from build123d import *

# Parameters (mm, degrees)
BOSS_EXTRUDE2_DEPTH = 3.175
SKETCH4_W           = 28.575
SKETCH4_H           = 79.375
CUT_EXTRUDE2_DEPTH  = 3.175
CUT_EXTRUDE3_DEPTH  = 3.175
SKETCH9_R           = 3.175
CUT_EXTRUDE4_DEPTH  = 3.175
SKETCH11_W          = 25.4
SKETCH11_H          = 3.175
BOSS_EXTRUDE3_DEPTH = 12.7
FILLET2_R           = 3.175


with BuildPart() as part:
    # Sketch1 → Boss-Extrude2 (new body)
    with BuildSketch(Plane.XY):
        Polygon((0, 298.45), (25.4, 323.85), (279.4, 323.85), (304.8, 298.45), (304.8, 25.4), (279.4, 0), (25.4, 0), (0, 25.4), align=None)
    extrude(amount=BOSS_EXTRUDE2_DEPTH)

    # Sketch4 → Cut-Extrude2 (cut)
    with BuildSketch(Plane.XY.offset(3.175)):
        with Locations((14.2875, 161.925)):
            Rectangle(SKETCH4_W, SKETCH4_H)
    extrude(amount=-CUT_EXTRUDE2_DEPTH, mode=Mode.SUBTRACT)

    # Sketch5 → Cut-Extrude3 (cut)
    with BuildSketch(Plane.XY.offset(3.175)):
        with BuildLine():
            Line((98.425, 275.149783319), (247.65, 275.149783319))
            ThreePointArc((247.65, 275.149783319), (270.100640303, 265.850423621), (279.4, 243.399783319))
            Line((279.4, 243.399783319), (279.4, 207.424891659))
            ThreePointArc((279.4, 207.424891659), (270.100640303, 184.974251357), (247.65, 175.674891659))
            Line((247.65, 175.674891659), (98.425, 175.674891659))
            ThreePointArc((98.425, 175.674891659), (75.974359697, 184.974251357), (66.675, 207.424891659))
            Line((66.675, 207.424891659), (66.675, 243.399783319))
            ThreePointArc((66.675, 243.399783319), (75.974359697, 265.850423621), (98.425, 275.149783319))
        make_face()
        with BuildLine():
            Line((98.425, 150.274891659), (247.65, 150.274891659))
            ThreePointArc((247.65, 150.274891659), (270.100640303, 140.975531962), (279.4, 118.524891659))
            Line((279.4, 118.524891659), (279.4, 82.55))
            ThreePointArc((279.4, 82.55), (270.100640303, 60.099359697), (247.65, 50.8))
            Line((247.65, 50.8), (98.425, 50.8))
            ThreePointArc((98.425, 50.8), (75.974359697, 60.099359697), (66.675, 82.55))
            Line((66.675, 82.55), (66.675, 118.524891659))
            ThreePointArc((66.675, 118.524891659), (75.974359697, 140.975531962), (98.425, 150.274891659))
        make_face()
    extrude(amount=-CUT_EXTRUDE3_DEPTH, mode=Mode.SUBTRACT)

    # Sketch9 → Cut-Extrude4 (cut)
    with BuildSketch(Plane.XY.offset(3.175)):
        with Locations((25.4, 301.625)):
            Circle(SKETCH9_R)
    extrude(amount=-CUT_EXTRUDE4_DEPTH, mode=Mode.SUBTRACT)

    # Sketch11 → Boss-Extrude3 (add)
    with BuildSketch(Plane.XY.offset(3.175)):
        with Locations((25.4, 296.8625)):
            Rectangle(SKETCH11_W, SKETCH11_H)
    extrude(amount=BOSS_EXTRUDE3_DEPTH)

    # Fillet2
    fillet2_edges = [part.edges().sort_by_distance(p)[0] for p in [
        (25.4, 295.275, 3.175),
    ]]
    fillet(fillet2_edges, radius=FILLET2_R)


solid = part.part
Input: part model. Units: mm. Frame: model coordinates. A direction names the side the tool comes from. Give positions to 0.01 mm unless a question says otherwise; leave off trailing zeros. Write each loop counter-clockwise with the first axis right and the second up, starting at its lowest first coordinate (ties: lowest second). Pieces come first, ordered by that corner, then holes.
Q1. Section C-C, the plane x = 264.5. Output: boundary loops of the cut face in (y, z) (3 decimals), plus the area to 3 significant figures.
Q2. First-contact query: P1, Ø7, axis at y = 296.5, z = 11.5, coming from the -X side; P2, Ø3, axis at y = 296, z = 11, coming from the +X side; P3, Ø1, axis at y = 174, z = 2, coming from the -X side (3 decimals); P4, Ø5.5, axis at x = 25.4, y = 301.625, coming from the +Z side. Flat tips, straight axial feed; report the tip coordinate or a pass-through.
Q3. Set-up query: faces 4 (the face through (25, 298.45, 9)), 5 (the face through (291.92, 311.33, 1.57)), 6 (the face through (12.9, 12.5, 1.6)), 7 (the face through (25, 295.275, 11)), 8 (the face through (270, 60, 2)). Return all of +Z, -Z, +X, -X, +Y, -Y with unobstructed straight access to the full face (end or side cutting, diameter ignored); none if empty.
Q4. Pull-direction query (X, two-part tool) for faces 1 (the face through (155, 164, 3.175)), 2 (the face through (76.22, 184.73, 1.61)), 3 (the face through (292.3, 12.9, 1.6)); classes: pulls with the +X half, pulls with the -X half, needs draft (parallel to the pull), parting line crosses it, or undercut.
Q5. Section D-D, the plane z = 13. Output: boundary loops of the cut face in (x, y) (3 decimals), plus the area to 3 significant figures.
Q6. Material intervals for probe 1 along Y at (x, z) = (25.4, 1.05); probe 2 along Y at (x, z) = (213.5, 2.5); probe 3 along Z at (x, y) = (69.5, 64) (3 decimals), sorted ascending.
Q7. Section B-B, the plane y = 63.5. Output: boundary loops of the cut face in (x, z) (3 decimals).
Q8. Section A-A, the plane x = 103.5. Output: boundary loops of the cut face in (y, z) (3 decimals), plus the area to 3 significant figures.
Filled in:
1. outline: (0, 0) - (55.64, 0) - (55.64, 3.175) - (0, 3.175) - close; (145.435, 0) - (180.515, 0) - (180.515, 3.175) - (145.435, 3.175) - close; (270.31, 0) - (323.85, 0) - (323.85, 3.175) - (270.31, 3.175) - close
1. area: 458 mm2
2. P1: stops at x = 12.7
2. P2: stops at x = 38.1
2. P3: stops at x = 28.575
2. P4: passes through
3. face 4: +Z, +X, -X, +Y
3. face 5: +Z, -Z, +X, +Y
3. face 6: +Z, -Z, -X, -Y
3. face 7: +Z, +X, -X, -Y
3. face 8: +Z, -Z
4. face 1: needs draft
4. face 2: undercut
4. face 3: pulls with the +X half
5. outline: (12.7, 295.275) - (38.1, 295.275) - (38.1, 298.45) - (12.7, 298.45) - close
5. area: 80.6 mm2
6. probe 1: y = 0 to 122.24, 201.61 to 298.45, 304.8 to 323.85
6. probe 2: y = 0 to 50.8, 150.27 to 175.67, 275.15 to 323.85
6. probe 3: z = 0 to 3.175
7. outline: (0, 0) - (73.025, 0) - (73.025, 3.175) - (0, 3.175) - close; (273.05, 0) - (304.8, 0) - (304.8, 3.175) - (273.05, 3.175) - close
8. outline: (0, 0) - (50.8, 0) - (50.8, 3.175) - (0, 3.175) - close; (150.275, 0) - (175.675, 0) - (175.675, 3.175) - (150.275, 3.175) - close; (275.15, 0) - (323.85, 0) - (323.85, 3.175) - (275.15, 3.175) - close
8. area: 397 mm2
